Can you work these out from the model? Positions are in its coordinate system, mm. A direction names the side the tool comes from. Round coordinates to 2 decimals unless told otherwise and drop trailing zeros. Order: outer loops, then holes, each group sorted by start corner. A loop starts at its lowest first (then second) coordinate and runs counter-clockwise, first axis right, second up.
from build123d import *

# Parameters (mm, degrees)
SWEEP2_PROFILE_R    = 5
SWEEP3_PROFILE_R    = 5
EXTRUDE_THIN2_DEPTH = 5
FILLET4_R           = 5
BOSS_EXTRUDE1_DEPTH = 1


with BuildPart() as part:
    # Sweep2: sweep along a path in Sketch14
    with BuildLine(Plane.XY) as sweep2_path:
        Line((-400, 0), (400, 0))
    # Sweep2 profile (on start of the path) → Sweep2 (sweep)
    with BuildSketch(Plane(origin=(-400, 0, 0), x_dir=(0, 0, 1), z_dir=(1, 0, 0))):
        Circle(SWEEP2_PROFILE_R)
    sweep(path=sweep2_path.line)



with BuildPart() as body_2:
    # Sweep3: sweep along a path in Sketch14<3>
    with BuildLine(Plane.XY) as sweep3_path:
        Line((-400, 300), (400, 300))
    # Sweep3 profile (on start of the path) → Sweep3 (sweep)
    with BuildSketch(Plane(origin=(-400, 300, 0), x_dir=(0, 0, 1), z_dir=(1, 0, 0))):
        Circle(SWEEP3_PROFILE_R)
    sweep(path=sweep3_path.line)


with BuildPart() as part_1:
    add(part.part)

    add(body_2.part)  # Extrude-Thin2 merges body 2
    # Sketch31 → Extrude-Thin2 (add, symmetric)
    with BuildSketch(Plane.XY):
        Polygon((400, -5), (400, 995), (-400, 995), (-400, -5), (-410, -5), (-410, 1005), (410, 1005), (410, -5), align=None)
    extrude(amount=EXTRUDE_THIN2_DEPTH, both=True)

    # Fillet4
    fillet4_edges = [part_1.edges().sort_by_distance(p)[0] for p in [
        (405, -5, -5),
        (405, -5, 5),
        (-410, -5, 0),
        (-405, -5, 5),
    ]]
    fillet(fillet4_edges, radius=FILLET4_R - 0.0001)  # a hair under: the kernel refuses the full size

    # Sketch32 → Boss-Extrude1 (add)
    with BuildSketch(Plane.XY):
        Polygon((275, 0), (275, 315), (-275, 315), (-275, 0), (-410, 0), (-410, 1005), (410, 1005), (410, 0), align=None)
    extrude(amount=BOSS_EXTRUDE1_DEPTH)


solid = part_1.part
(1) I'm going to push flat-ended pins straight in: pin 1 Ø1.2 at (x, z) = (188, 2.5) entering from -Y; pin 2 Ø4 at (x, z) = (134.5, -3) entering from -Y; pin 3 Ø5 at (x, y) = (324, 677.5) entering from +Z. Where does each tip first touch, or does it pass through?
(2) I want a section at D-D, the plane y = 657.5. List the corners of the cut face in (x, z) for me, plus the area to 3 significant figures.
(3) I want a section at C-C, the plane z = -1.75. Give the number of separate pieces and of enclosed holes in the cut face, plus the area to 3 significant figures.
(4) Please list where these lines run through material, in increasing order: probe 1 along Y at (x, z) = (146.5, 0.5); probe 2 along Y at (x, z) = (-88.5, -1.5); probe 3 along X at (y, z) = (712.5, 2.75).
(5) On a 3-axis mill with a long thin cutter (end or side, diameter ignored), from which of +Z, -Z, +X, -X, +Y, -Y can I reach the whole of each face in a straight line? I mean faces 3 (the face through (6, 655, 1)), 4 (the face through (-337, 152, 0)). Say none if no direction works.
(6) I want a section at B-B, the plane y = 125. List the corners of the cut face in (x, z) for me, plus the area to 3 significant figures.
(7) I want a section at A-A, the plane x = -230. List the corners of the cut face in (y, z) for me, plus the area to 3 significant figures.
(8) If we mould it in two halves opening along X, with no side actions, what happens to faces 1 (the face through (338, 152, 0)), 2 (the face through (-337, 152, 1))? For each: pulls with the +X half, pulls with the -X half, needs draft (parallel to the pull), parting line crosses it, or undercut.
Ans:
1. pin 1: stops at y = -4.62
1. pin 2: stops at y = -4.9
1. pin 3: stops at z = 1
2. outline: (-410, -5) - (-400, -5) - (-400, 0) - (400, 0) - (400, -5) - (410, -5) - (410, 5) - (400, 5) - (400, 1) - (-400, 1) - (-400, 5) - (-410, 5) - close
2. area: 1,000 mm2
3. separate pieces: 1
3. enclosed holes: 2
3. area: 43,200 mm2
4. probe 1: y = -4.97 to 4.97, 295.03 to 304.97, 315 to 1005
4. probe 2: y = -4.77 to 4.77, 295.23 to 304.77, 995 to 1005
4. probe 3: x = -410 to -400, 400 to 410
5. face 3: +Z
5. face 4: -Z
6. outline: (-410, -5) - (-400, -5) - (-400, 0) - (-275, 0) - (-275, 1) - (-400, 1) - (-400, 5) - (-410, 5) - close; (275, 0) - (400, 0) - (400, -5) - (410, -5) - (410, 5) - (400, 5) - (400, 1) - (275, 1) - close
6. area: 450 mm2
7. outline: circle Ø10 at (0, 0); circle Ø10 at (300, 0); (315, 0) - (995, 0) - (995, -5) - (1005, -5) - (1005, 5) - (995, 5) - (995, 1) - (315, 1) - close
7. area: 937 mm2
8. face 1: undercut
8. face 2: undercut
